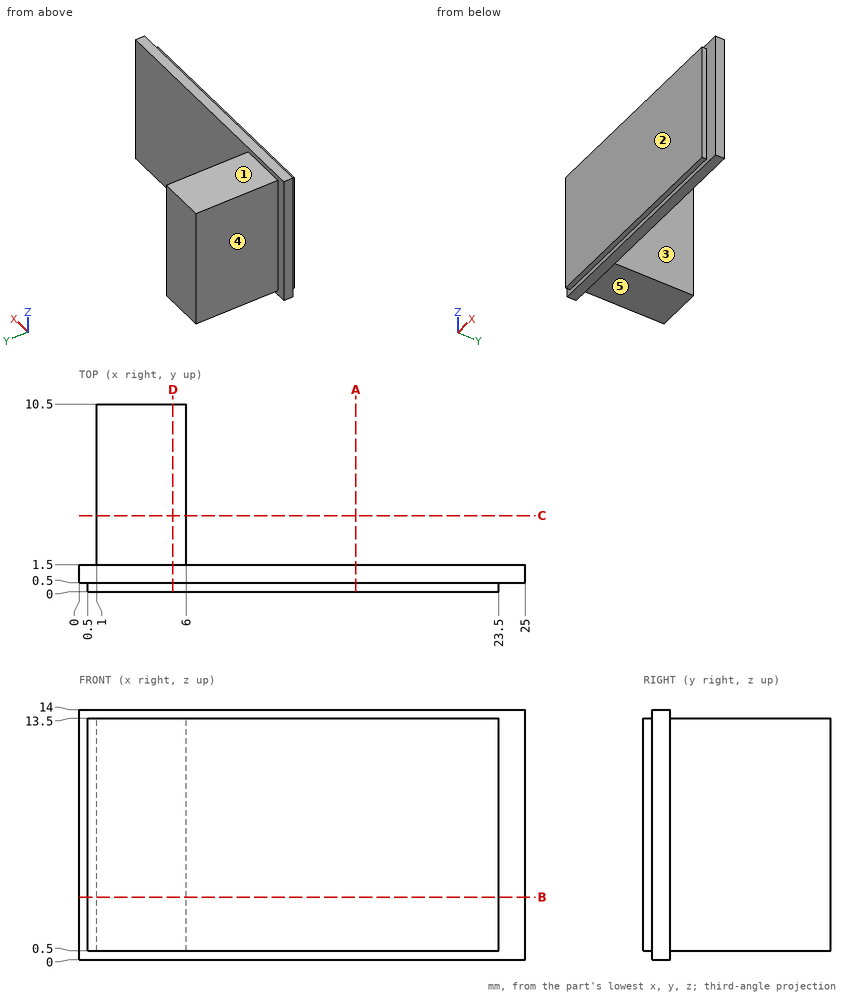
Check sheet for the drawn part. Datum: minimum x, y, z corner. Units: mm. A direction names the side the tool comes from. Coordinates: 2 decimals unless noted, no trailing zeros. Loops run counter-clockwise (first coordinate to the right, second up) from the corner with the lowest first, then second, coordinate; pieces in that order, holes last. Notation, with made-up numbers: (65, 23.5) -> (89, 23.5) arc R26 cw to (89, 47.5) -> close; hole circle Ø11 at (40, 19). An arc over 180 degrees is marked (long way). Write each question's results on one line, items separated by ' | '.
Item 1: Material ranges on L1, parallel to Y at x = 10.25, z = 11.25; L2, parallel to Z at x = 2.25, y = 7.5; L3, parallel to X at y = 4, z = 7, recorded low to high.
Found:
L1: y = 0 to 1.5 | L2: z = 0.5 to 13.5 | L3: x = 1 to 6
Item 2: Gauge pin test, flat ends, axial feed: pin 1 (1.5 mm diameter, centred on x = 4.5, y = 5, fed in from +Z); pin 2 (0.6 mm diameter, centred on y = 0, z = 6.5, fed in from -X); pin 3 (1 mm diameter, centred on x = 3.5, z = 3.5, fed in from -Y); pin 4 (4 mm diameter, centred on x = 16, z = 5.5, fed in from +Y). Record the tip position at first contact, or that the pin passes through.
Found:
pin 1: stops at z = 13.5 | pin 2: stops at x = 0.5 | pin 3: stops at y = 0 | pin 4: stops at y = 1.5
Item 3: Section check B-B, the plane z = 3.5. Enter the section's corners in (x, y), plus the area to 3 significant figures.
Found:
outline: (0, 0.5) -> (0.5, 0.5) -> (0.5, 0) -> (23.5, 0) -> (23.5, 0.5) -> (25, 0.5) -> (25, 1.5) -> (6, 1.5) -> (6, 10.5) -> (1, 10.5) -> (1, 1.5) -> (0, 1.5) -> close | area: 81.5 mm2
Item 4: Section check A-A, the plane x = 15.5. Enter the section's corners in (y, z), plus the area to 3 significant figures.
Found:
outline: (0, 0.5) -> (0.5, 0.5) -> (0.5, 0) -> (1.5, 0) -> (1.5, 14) -> (0.5, 14) -> (0.5, 13.5) -> (0, 13.5) -> close | area: 20.5 mm2
Item 5: Tool access check on the marked faces 1, 2, 3, 4 and 5. Record the directions out of +Z, -Z, +X, -X, +Y, -Y that give a thin tool (end or side, any length) a straight path to the whole face; none if there is none.
Found:
face 1: +Z, +X, -X, +Y | face 2: +Z, -Z, +X, -X, -Y | face 3: +Z, -Z, +X, +Y | face 4: +Z, -Z, -X, +Y | face 5: -Z, +X, -X, +Y
Item 6: Section check C-C, the plane y = 4.25. Enter the section's corners in (x, z).
Found:
outline: (1, 0.5) -> (6, 0.5) -> (6, 13.5) -> (1, 13.5) -> close
Item 7: Section check D-D, the plane x = 5.25. Enter the section's corners in (y, z).
Found:
outline: (0, 0.5) -> (0.5, 0.5) -> (0.5, 0) -> (1.5, 0) -> (1.5, 0.5) -> (10.5, 0.5) -> (10.5, 13.5) -> (1.5, 13.5) -> (1.5, 14) -> (0.5, 14) -> (0.5, 13.5) -> (0, 13.5) -> close
